Read the model definition and answer for the solid it produces. Units are mm, in the model's axes. Give positions to 0.01 mm unless a question says otherwise; leave off trailing zeros. Write each loop counter-clockwise with the first axis right and the second up, starting at its lowest first coordinate (ties: lowest second). Pieces come first, ordered by that corner, then holes. Notation, with made-up numbers: M -15.75,-36.5 L -9.75,-36.5 A29 ccw -9.75,-9.5 Z; hole C 77,49.25 d11. An arc over 180 degrees is marked long. Use a Markdown table: item, result. Add a question column.
Item 1: A cutting plane is placed at A-A on x = 7.75. Determine the outline of the cut face in (y, z), then the cut area to 3 significant figures.
Item 2: Consider probe 1 along Y at (x, z) = (8, 1.4); probe 2 along Z at (x, y) = (-1.75, -7.5); probe 3 along Y at (x, z) = (0.5, 1.8). Determine where each line is inside the solid, lowest interval first. Write a range as [from, to].
Item 3: A cutting plane is placed at C-C on x = 1.5. Determine the outline of the cut face in (y, z), then the cut area to 3 significant figures.
Item 4: A cutting plane is placed at D-D on z = 1. Determine the outline of the cut face in (x, y).
Item 5: A cutting plane is placed at B-B on y = 8.5. Determine the outline of the cut face in (x, z), then the cut area to 3 significant figures.
Item 6: Given P1, Ø3.5, axis at x = 7.747, y = 7.747, coming from the +Z side; P2, Ø1.6, axis at x = 0, z = 2.5, coming from the -Y side, each flat-ended and moving along its own axis, determine where each tip first touches the part or whether it passes through.
from build123d import *

# Parameters (mm, degrees)
SKETCH_1_W      = 20.066
SKETCH_1_H      = 20.066
SKETCH_1_R      = 1.6
EXTRUDE_1_DEPTH = 1.5
SKETCH_2_W      = 4
SKETCH_2_H      = 4
EXTRUDE_2_DEPTH = 1.5


with BuildPart() as part:
    # 草图1 → 凸台-拉伸1 (new body)
    with BuildSketch(Plane.XY):
        Rectangle(SKETCH_1_W, SKETCH_1_H)
        with Locations((-7.747, 7.747)):
            Circle(SKETCH_1_R, mode=Mode.SUBTRACT)
        with Locations((7.747, 7.747)):
            Circle(SKETCH_1_R, mode=Mode.SUBTRACT)
        with Locations((-7.747, -7.747)):
            Circle(SKETCH_1_R, mode=Mode.SUBTRACT)
        with Locations((7.747, -7.747)):
            Circle(SKETCH_1_R, mode=Mode.SUBTRACT)
    extrude(amount=EXTRUDE_1_DEPTH)

    # 草图2 → 凸台-拉伸2 (add)
    with BuildSketch(Plane.XY.offset(1.5)):
        Rectangle(SKETCH_2_W, SKETCH_2_H)
    extrude(amount=EXTRUDE_2_DEPTH)


solid = part.part
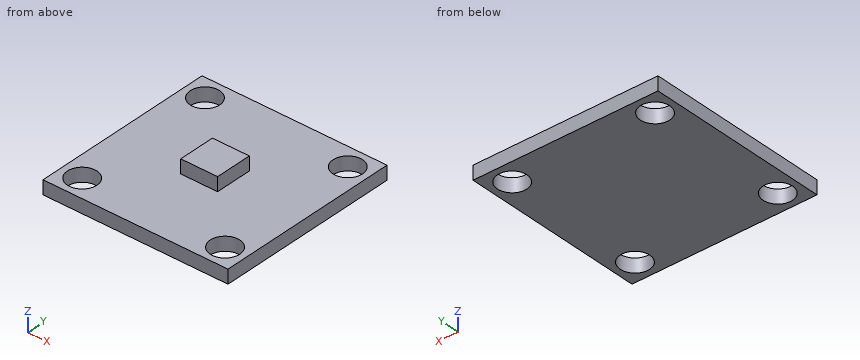
Filled in:
| question | item | result |
|---|---|---|
| 1 | outline | M -10.03,0 L -9.35,0 L -9.35,1.5 L -10.03,1.5 Z; M -6.15,0 L 6.15,0 L 6.15,1.5 L -6.15,1.5 Z; M 9.35,0 L 10.03,0 L 10.03,1.5 L 9.35,1.5 Z |
| 1 | area | 20.5 mm² |
| 2 | probe 1 | [-10.03, -9.33], [-6.17, 6.17], [9.33, 10.03] |
| 2 | probe 2 | [0, 1.5] |
| 2 | probe 3 | [-2, 2] |
| 3 | outline | M -10.03,0 L 10.03,0 L 10.03,1.5 L 2,1.5 L 2,3 L -2,3 L -2,1.5 L -10.03,1.5 Z |
| 3 | area | 36.1 mm² |
| 4 | outline | M -10.03,-10.03 L 10.03,-10.03 L 10.03,10.03 L -10.03,10.03 Z; hole C -7.75,-7.75 d3.2; hole C -7.75,7.75 d3.2; hole C 7.75,-7.75 d3.2; hole C 7.75,7.75 d3.2 |
| 5 | outline | M -10.03,0 L -9.16,0 L -9.16,1.5 L -10.03,1.5 Z; M -6.34,0 L 6.34,0 L 6.34,1.5 L -6.34,1.5 Z; M 9.16,0 L 10.03,0 L 10.03,1.5 L 9.16,1.5 Z |
| 5 | area | 21.6 mm² |
| 6 | P1 | z = 1.5 |
| 6 | P2 | y = -2 |
